```python
from build123d import *

# Parameters (mm, degrees)
BOSS_EXTRUDE1_DEPTH                             = 15
CHAMFER1_SIZE                                   = 2.5
SKETCH2_R                                       = 1.4
CUT_EXTRUDE1_DEPTH                              = 15
CHAMFER2_SIZE                                   = 2
SKETCH3_R                                       = 1.4
CUT_EXTRUDE2_DEPTH                              = 47.129659115
CUT_EXTRUDE3_DEPTH                              = 25
CSK_FOR_M3_FLAT_HEAD_MACHINE_SCREW1_D           = 3
CSK_FOR_M3_FLAT_HEAD_MACHINE_SCREW1_DEPTH       = 31.098709071
CSK_FOR_M3_FLAT_HEAD_MACHINE_SCREW1_CSINK_D     = 6.3
CSK_FOR_M3_FLAT_HEAD_MACHINE_SCREW1_CSINK_ANGLE = 90
CSK_FOR_M3_FLAT_HEAD_MACHINE_SCREW1_TIP         = 0.901290929


with BuildPart() as part:
    # Sketch1 → Boss-Extrude1 (new body)
    with BuildSketch(Plane.XY):
        with BuildLine():
            Line((-19, 0), (-19, -4))
            Line((-19, -4), (-34, -4))
            Line((-34, -4), (-34, 0))
            Line((-34, 0), (-22.883234523, 0))
            ThreePointArc((-22.883234523, 0), (-17.861391251, 14.304304416), (-5, 22.33030278))
            Line((-5, 22.33030278), (-5, 27.33030278))
            Line((-5, 27.33030278), (-1, 27.33030278))
            Line((-1, 27.33030278), (-1, 18.33030278))
            Line((-1, 18.33030278), (-5, 18.33030278))
            ThreePointArc((-5, 18.33030278), (-15.099668871, 11.532562595), (-19, 0))
        make_face()
    extrude(amount=BOSS_EXTRUDE1_DEPTH)

    # Chamfer1
    chamfer1_edges = [part.edges().sort_by_distance(p)[0] for p in [
        (-34, -2, 0),
        (-34, -2, 15),
    ]]
    chamfer(chamfer1_edges, length=CHAMFER1_SIZE)

    # Sketch2 → Cut-Extrude1 (cut)
    with BuildSketch(Plane.ZY.offset(5)):
        with Locations(Location((2.8, 24.83030278, 0), (0, 0, 270))):
            Circle(SKETCH2_R)
        with Locations(Location((12.2, 24.83030278, 0), (0, 0, 270))):
            Circle(SKETCH2_R)
    extrude(amount=-CUT_EXTRUDE1_DEPTH, mode=Mode.SUBTRACT)

    # Chamfer2
    chamfer2_edges = [part.edges().sort_by_distance(p)[0] for p in [
        (-3, 27.33030278, 0),
        (-3, 27.33030278, 15),
    ]]
    chamfer(chamfer2_edges, length=CHAMFER2_SIZE)

    # Sketch3 → Cut-Extrude2 (cut, through all)
    with BuildSketch(Plane(origin=(0, 0, 0), x_dir=(1, 0, 0), z_dir=(0, 1, 0))):
        with Locations(Location((-28.441617262, -7.5, 0), (0, 0, 270))):
            Circle(SKETCH3_R)
    extrude(amount=-CUT_EXTRUDE2_DEPTH, mode=Mode.SUBTRACT)

    # Sketch4 → Cut-Extrude3 (cut)
    with BuildSketch(Plane.XZ.offset(4)):
        Polygon((-24.636069701, 0), (-34, 6.600391812), (-34, 2.5), (-31.5, 0), align=None)
    extrude(amount=-CUT_EXTRUDE3_DEPTH, mode=Mode.SUBTRACT)

    # CSK for M3 Flat Head Machine Screw1
    with Locations(Plane(origin=(0, 0, 0), x_dir=(1, 0, 0), z_dir=(0, 1, 0))):
        with Locations((-28.441617262, -7.5)):
            CounterSinkHole(CSK_FOR_M3_FLAT_HEAD_MACHINE_SCREW1_D / 2, CSK_FOR_M3_FLAT_HEAD_MACHINE_SCREW1_CSINK_D / 2, depth=CSK_FOR_M3_FLAT_HEAD_MACHINE_SCREW1_DEPTH, counter_sink_angle=CSK_FOR_M3_FLAT_HEAD_MACHINE_SCREW1_CSINK_ANGLE)
            with Locations((0, 0, -(CSK_FOR_M3_FLAT_HEAD_MACHINE_SCREW1_DEPTH + CSK_FOR_M3_FLAT_HEAD_MACHINE_SCREW1_TIP / 2))):  # 118° drill point
                Cone(0, CSK_FOR_M3_FLAT_HEAD_MACHINE_SCREW1_D / 2, CSK_FOR_M3_FLAT_HEAD_MACHINE_SCREW1_TIP, mode=Mode.SUBTRACT)


solid = part.part
```
Model file for the job. Use its own axes, mm. A direction names the side the tool comes from. Give positions to 0.01 mm unless a question says otherwise; leave off trailing zeros. Loops run counter-clockwise (first coordinate to the right, second up) from the corner with the lowest first, then second, coordinate; pieces in that order, holes last. Notation, with made-up numbers: (53.25, -6) -> (105.25, -6) arc R24 ccw to (105.25, 4) -> close; hole circle Ø3 at (81.25, 12). An arc over 180 degrees is marked (long way). Write each question's results on one line, items separated by ' | '.
(1) Flat gauge pins, fed straight in: pin 1 Ø3.5 at (y, z) = (24.83, 2.8) entering from -X; pin 2 Ø8 at (x, y) = (-22, 17) entering from +Z; pin 3 Ø3 at (y, z) = (3.5, 11) entering from -X; pin 4 Ø6 at (x, z) = (-19.5, 5.5) entering from +Y. Where does each tip first touch, or does it go through?
Geometry results:
pin 1: stops at x = -5 | pin 2: passes through | pin 3: stops at x = -22.8 | pin 4: stops at y = 15.86
(2) Cut at D-D on x = -7. List the corners of the cut face in (y, z).
Geometry results:
outline: (17.66, 0) -> (21.79, 0) -> (21.79, 15) -> (17.66, 15) -> close
(3) Cut at A-A on z = 7.5. List the corners of the cut face in (x, y), and give its area (3 significant figures).
Geometry results:
outline: (-34, -4) -> (-29.94, -4) -> (-29.94, -1.65) -> (-31.59, 0) -> (-34, 0) -> close; (-26.94, -4) -> (-19, -4) -> (-19, 0) arc R19 cw to (-5, 18.33) -> (-1, 18.33) -> (-1, 27.33) -> (-5, 27.33) -> (-5, 22.33) arc R22.88 ccw to (-22.88, 0) -> (-25.29, 0) -> (-26.94, -1.65) -> close | area: 189 mm²
(4) Cut at C-C on y = 17. List the corners of the cut face in (x, z), and give its area (3 significant figures).
Geometry results:
outline: (-15.32, 0) -> (-8.49, 0) -> (-8.49, 15) -> (-15.32, 15) -> close | area: 102 mm²
(5) Probe line 1 along X through (y, z) = (-2.25, 7.5); line 2 along Y through (x, z) = (-23, 0.75); line 3 along X through (y, z) = (26, 5). List the from-to ranges inside material, lowest first.
Geometry results:
line 1: x = -34 to -29.94, -26.94 to -19 | line 2: y = -4 to 0 | line 3: x = -5 to -1
(6) Cut at B-B on z = 2.8. List the corners of the cut face in (x, y), and give its area (3 significant figures).
Geometry results:
outline: (-28.61, -4) -> (-19, -4) -> (-19, 0) arc R19 cw to (-5, 18.33) -> (-1, 18.33) -> (-1, 23.43) -> (-5, 23.43) -> (-5, 22.33) arc R22.88 ccw to (-22.88, 0) -> (-28.61, 0) -> close; (-5, 26.23) -> (-1, 26.23) -> (-1, 27.33) -> (-5, 27.33) -> close | area: 171 mm²
(7) Pull direction X, two halves, no side cores. Call faces 4 (the cylindrical face through (-26.943, -2.841, 7.434)), 5 (the flat face through (-3.03, 26.34, 1.01)), 6 (the flat face through (-34, -2, 10)): released by +X, released by -X, zero draft, split by the parting line, or undercut.
Geometry results:
face 4: undercut | face 5: zero draft | face 6: released by -X
(8) Tool access for faces 1 (the flat face through (-1, 23, 7)), 2 (the flat face through (-27, 0, 11)), 3 (the flat face through (-19, -2, 7)): list every direction of +Z, -Z, +X, -X, +Y, -Y with a clear straight run to the whole face (end or side of a thin tool).
Geometry results:
face 1: +Z, -Z, +X, +Y, -Y | face 2: +Z, -Z, -X, +Y | face 3: +Z, -Z, +X, -Y
